```python
from build123d import *

# Parameters (mm, degrees)
BOSS_EXTRUDE2_DEPTH = 10
SKETCH2_R           = 2.5
CUT_EXTRUDE1_DEPTH  = 10


with BuildPart() as part:
    # Sketch1 → Boss-Extrude2 (new body)
    with BuildSketch(Plane.XY):
        with BuildLine():
            Line((-12.770888736, 48.650584459), (-12.770888736, -21.349415541))
            ThreePointArc((-12.770888736, -21.349415541), (-13.250610219, -29.329137023), (-5.270888736, -28.849415541))
            Line((-5.270888736, -28.849415541), (64.729111264, -28.849415541))
            Line((64.729111264, -28.849415541), (64.729111264, -21.349415541))
            Line((64.729111264, -21.349415541), (-5.270888736, -21.349415541))
            Line((-5.270888736, -21.349415541), (-5.270888736, 48.650584459))
            Line((-5.270888736, 48.650584459), (-12.770888736, 48.650584459))
        make_face()
    extrude(amount=BOSS_EXTRUDE2_DEPTH)

    # Sketch2 → Cut-Extrude1 (cut)
    with BuildSketch(Plane(origin=(0, 0, 0), x_dir=(-1, 0, 0), z_dir=(0, 0, -1))):
        with Locations((9.47340598, -25.551932785)):
            Circle(SKETCH2_R)
    extrude(amount=-CUT_EXTRUDE1_DEPTH, mode=Mode.SUBTRACT)


solid = part.part
```
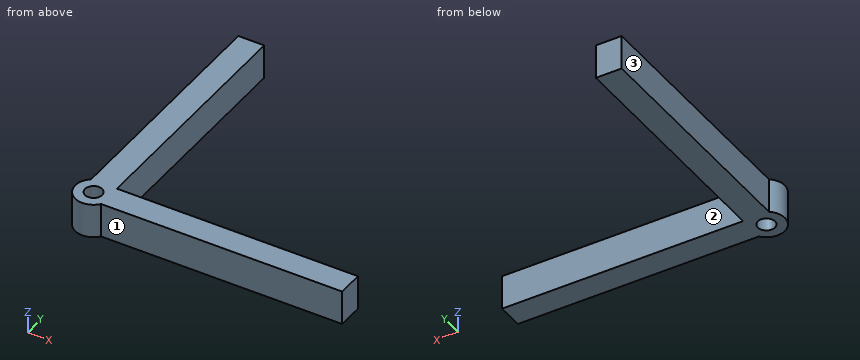
Here's how the part is built. I have some questions about the finished solid (model axes, mm). Face numbers are marked on the shaded views. A direction names the side the tool comes from. Coordinates: 2 decimals unless noted, no trailing zeros. Order: outer loops, then holes, each group sorted by start corner. A loop starts at its lowest first (then second) coordinate and runs counter-clockwise, first axis right, second up.
Item 1: I'm going to push flat-ended pins straight in: pin 1 Ø2 at (x, z) = (38, 1.5) entering from +Y; pin 2 Ø2 at (y, z) = (22.5, 7.5) entering from +X; pin 3 Ø1 at (y, z) = (-11, 6.5) entering from -X. Where does each tip first touch, or does it pass through?
Response values:
pin 1: stops at y = -21.35
pin 2: stops at x = -5.27
pin 3: stops at x = -12.77
Item 2: I need wall thicknesses on probe 1 along X at (y, z) = (-7.5, 4.5); probe 2 along Y at (x, z) = (3, 3); probe 3 along Y at (x, z) = (-10.5, 8.5). Which ranges of each line are inside material? Lowest first, please.
Response values:
probe 1: x = -12.77 to -5.27
probe 2: y = -28.85 to -21.35
probe 3: y = -30.79 to -27.83, -23.27 to 48.65
Item 3: If we section it at B-B, the plane x = 9.5: List the corners of the cut face in (y, z) for me.
Response values:
outline: (-28.85, 0) - (-21.35, 0) - (-21.35, 10) - (-28.85, 10) - close
Item 4: If we section it at C-C, the plane y = 37.5: List the corners of the cut face in (x, z) for me.
Response values:
outline: (-12.77, 0) - (-5.27, 0) - (-5.27, 10) - (-12.77, 10) - close
Item 5: If we section it at A-A, the plane z = 2.75: List the corners of the cut face in (x, y) for me, then the cut area to 3 significant figures.
Response values:
outline: (-12.77, -21.35) arc R5.34 ccw (long way) to (-5.27, -28.85) - (64.73, -28.85) - (64.73, -21.35) - (-5.27, -21.35) - (-5.27, 48.65) - (-12.77, 48.65) - close; hole circle Ø5 at (-9.47, -25.55)
area: 1,110 mm2
Item 6: Which directions (+Z, -Z, +X, -X, +Y, -Y) give clear straight access to the entire face, cutting with the end or side of a thin tool? Please do the marked faces 1, 2 and 3.
Response values:
face 1: +Z, -Z, +X, -Y
face 2: +Z, -Z, +X, +Y
face 3: +Z, -Z, -X, +Y
